from build123d import *

# Parameters (mm, degrees)
SKETCH1_W           = 152.4
SKETCH1_H           = 25.4
BOSS_EXTRUDE1_DEPTH = 6.35
SKETCH3_W           = 6.35
SKETCH3_H           = 12.7
BOSS_EXTRUDE2_DEPTH = 6.35


with BuildPart() as part:
    # Sketch1 → Boss-Extrude1 (new body)
    with BuildSketch(Plane(origin=(0, 0, 0), x_dir=(1, 0, 0), z_dir=(0, 1, 0))):
        with Locations((76.2, -12.7)):
            Rectangle(SKETCH1_W, SKETCH1_H)
    extrude(amount=BOSS_EXTRUDE1_DEPTH)

    # Sketch3 → Boss-Extrude2 (add)
    with BuildSketch(Plane(origin=(0, 6.35, 0), x_dir=(1, 0, 0), z_dir=(0, 1, 0))):
        with Locations((-3.175, -12.7)):
            Rectangle(SKETCH3_W, SKETCH3_H)
    boss_extrude2 = extrude(amount=-BOSS_EXTRUDE2_DEPTH)

    # Mirror1: Boss-Extrude2 across plane
    add(boss_extrude2.mirror(Plane.ZY.offset(-76.2)))


solid = part.part
Input: part model. Units: mm. Frame: model coordinates. A direction names the side the tool comes from. Give positions to 0.01 mm unless a question says otherwise; leave off trailing zeros. Loops run counter-clockwise (first coordinate to the right, second up) from the corner with the lowest first, then second, coordinate; pieces in that order, holes last. Notation, with made-up numbers: (-10, -3) -> (14, -3) arc R15 cw to (14, 8) -> close; hole circle Ø3 at (18.25, 72.5). An arc over 180 degrees is marked (long way). Answer as a JSON object with one key per item and string values. Group by question number.
Item 1: Cut plane A-A, the plane y = 5.25. Return the cut outline in (x, z).
Item 2: Pin query (flat end, axial travel): P1, Ø1.9, axis at x = 155.5, y = 2.5, coming from the -Z side; P2, Ø3, axis at y = 2.5, z = 22, coming from the -X side; P3, Ø3, axis at y = 4, z = 2, coming from the +X side. Return the tip coordinate at first contact, or that it passes through.
Item 3: Line query: probe 1 along X at (y, z) = (2.75, 20.25). Output: solid intervals per line, ascending.
Item 4: Reachability of faces 1 (the flat face through (156, 3, 6.35)), 2 (the flat face through (0, 3, 22)), 3 (the flat face through (152.4, 3, 22)) from +Z, -Z, +X, -X, +Y, -Y: full face, straight path, thin tool, end or side. Return the list, or none.
Item 5: Cut plane B-B, the plane z = 4.5. Return the cut outline in (x, y), and give its area (3 significant figures).
Checks:
{
 "1": {"outline": "(-6.35, 6.35) -> (0, 6.35) -> (0, 0) -> (152.4, 0) -> (152.4, 6.35) -> (158.75, 6.35) -> (158.75, 19.05) -> (152.4, 19.05) -> (152.4, 25.4) -> (0, 25.4) -> (0, 19.05) -> (-6.35, 19.05) -> close"},
 "2": {"P1": "stops at z = 6.35", "P2": "stops at x = 0", "P3": "stops at x = 152.4"},
 "3": {"probe 1": "x = 0 to 152.4"},
 "4": {"face 1": "-Z, +X, +Y, -Y", "face 2": "+Z, -X, +Y, -Y", "face 3": "+Z, +X, +Y, -Y"},
 "5": {"outline": "(0, 0) -> (152.4, 0) -> (152.4, 6.35) -> (0, 6.35) -> close", "area": "968 mm²"}
}
